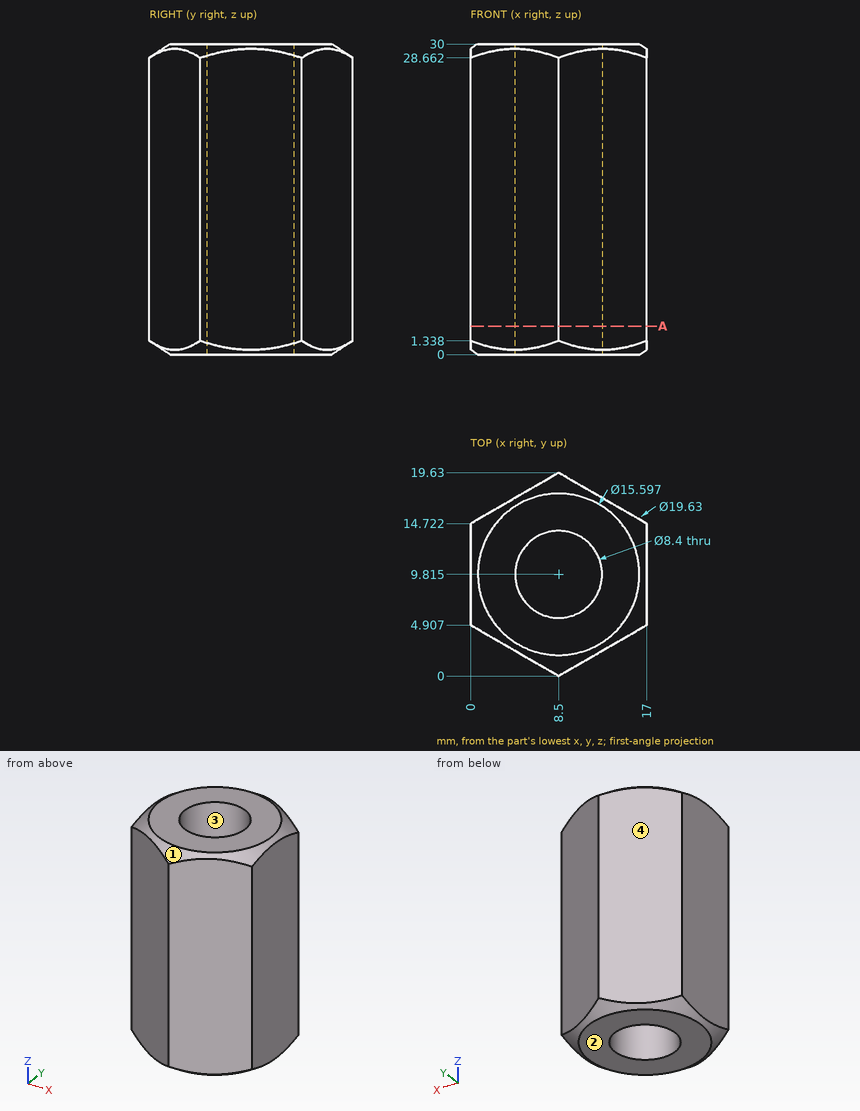
Check sheet for the drawn part. Datum: minimum x, y, z corner. Units: mm. Round coordinates to 2 decimals unless told otherwise and drop trailing zeros. Order: outer loops, then holes, each group sorted by start corner. A loop starts at its lowest first (then second) coordinate and runs counter-clockwise, first axis right, second up. Notation, with made-up numbers: (66, 41.25) -> (81, 41.25) arc R28 ccw to (81, 59.25) -> close; hole circle Ø7 at (2.25, 33). An arc over 180 degrees is marked (long way). Return JSON: item names as keys, results as strings. Group by question number.
Q1. Gauge pin test, flat ends, axial feed: pin 1 (1 mm diameter, centred on x = 5, z = 3.5, fed in from +Y); pin 2 (5 mm diameter, centred on x = 10, z = 3.5, fed in from -Y). Record the tip position at first contact, or that the pin passes through.
Q2. Release check for a two-part mould opening along X. For the marked faces 1, 2, 3 and 4 record: released by +X, released by -X, zero draft, split by the parting line, or undercut.
Q3. Section check A-A, the plane z = 2.75. Record the boundary of the cut face in (x, y) (1 decimal), plus the area to 3 significant figures.
Q4. Material ranges on probe 1 along X at (y, z) = (8.75, 16.5); probe 2 along X at (y, z) = (9.75, 21.75); probe 3 along Y at (x, z) = (11.25, 28.75), recorded low to high. Write a range as from..to.
Numbers:
{
 "1": {"pin 1": "y = 17.9", "pin 2": "y = 0"},
 "2": {"face 1": "split by the parting line", "face 2": "zero draft", "face 3": "undercut", "face 4": "released by -X"},
 "3": {"outline": "(0, 4.9) -> (8.5, 0) -> (17, 4.9) -> (17, 14.7) -> (8.5, 19.6) -> (0, 14.7) -> close; hole circle Ø8.4 at (8.5, 9.8)", "area": "195 mm^2"},
 "4": {"probe 1": "0..4.44, 12.56..17", "probe 2": "0..4.3, 12.7..17", "probe 3": "1.59..6.64, 12.99..18.04"}
}
